```python
from build123d import *

# Parameters (mm, degrees)
SKETCH2_R           = 8.626283366
SKETCH2_R_2         = 2
BOSS_EXTRUDE2_DEPTH = 0.15


with BuildPart() as part:
    # Sketch1 → Revolve1 (revolve)
    with BuildSketch(Plane.XY, mode=Mode.PRIVATE) as revolve1_sk:
        with BuildLine():
            Line((16, 21.11), (16, 20.123658445))
            ThreePointArc((16, 20.123658445), (14.844631277, 19.923379665), (14, 19.11))
            Line((14, 19.11), (14, 13.11))
            ThreePointArc((14, 13.11), (12.760912849, 9.212301981), (9.498573932, 6.745617646))
            ThreePointArc((9.498573932, 6.745617646), (8.602056269, 5.471944767), (7.096455966, 5.073003354))
            ThreePointArc((7.096455966, 5.073003354), (4.361623846, 1.398669209), (0, 0))
            Line((0, 0), (0, 20.221919192))
            ThreePointArc((0, 20.221919192), (5.230275248, 18.600523967), (8.626283366, 14.304964573))
            Line((8.626283366, 14.304964573), (8.626283366, 21.11))
            Line((8.626283366, 21.11), (16, 21.11))
        make_face()
    revolve(revolve1_sk.sketch.rotate(Axis((0, 20.221919192, 0), (0, -1, 0)), 90), axis=Axis((0, 20.221919192, 0), (0, -1, 0)))

    # Sketch2 → Boss-Extrude2 (add)
    with BuildSketch(Plane(origin=(0, 21.11, 0), x_dir=(1, 0, 0), z_dir=(0, 1, 0))):
        with BuildLine():
            Line((-4.400679072, -22.153645833), (-13.285068895, -8.916666667))
            ThreePointArc((-13.285068895, -8.916666667), (-16, 0), (-13.285068895, 8.916666667))
            Line((-13.285068895, 8.916666667), (-4.400679072, 22.153645833))
            ThreePointArc((-4.400679072, 22.153645833), (0, 24.5), (4.400679072, 22.153645833))
            Line((4.400679072, 22.153645833), (13.285068895, 8.916666667))
            ThreePointArc((13.285068895, 8.916666667), (16, 0), (13.285068895, -8.916666667))
            Line((13.285068895, -8.916666667), (4.400679072, -22.153645833))
            ThreePointArc((4.400679072, -22.153645833), (0, -24.5), (-4.400679072, -22.153645833))
        make_face()
        with Locations(Location((0, 0, 0), (0, 0, 270))):
            Circle(SKETCH2_R, mode=Mode.SUBTRACT)
        with Locations(Location((0, -19.2, 0), (0, 0, 270))):
            Circle(SKETCH2_R_2, mode=Mode.SUBTRACT)
        with Locations(Location((0, 19.2, 0), (0, 0, 270))):
            Circle(SKETCH2_R_2, mode=Mode.SUBTRACT)
    extrude(amount=BOSS_EXTRUDE2_DEPTH)


solid = part.part
```
Here's how the part is built. I have some questions about the finished solid (model axes, mm). Round coordinates to 2 decimals unless told otherwise and drop trailing zeros. Order: outer loops, then holes, each group sorted by start corner. A loop starts at its lowest first (then second) coordinate and runs counter-clockwise, first axis right, second up. Notation, with made-up numbers: (-4.75, 20) -> (6.25, 20) arc R21 ccw to (6.25, 28) -> close; hole circle Ø7 at (73.5, 57.25). An arc over 180 degrees is marked (long way). Use a Markdown table: item, result. Add a question column.
(1) I need wall thicknesses on line 1 along Z through (x, y) = (-6, 15.25); line 2 along X through (y, z) = (19.5, 0); line 3 along Z through (x, y) = (-7.5, 15). Which ranges of each line are inside material? Lowest first, please.
(2) For pin 1 Ø1.5 at (x, y) = (11.5, 12.5) entering from +Z; pin 2 Ø15.5 at (x, z) = (0, 0) entering from +Y; pin 3 Ø1 at (y, z) = (13.5, 0.5) entering from +X, each with a flat end and sliding along its axis, tell me the tip position at first contact or that it passes through.
(3) Suppose I cut it at D-D, the plane y = 15.5. Please give me the cut outline in (x, z).
(4) Suppose I cut it at C-C, the plane z = 0. Please give me the cut outline in (x, y).
(5) Suppose I cut it at B-B, the plane x = 0. Please give me the cut outline in (y, z), and give its area (3 significant figures).
(6) Suppose I cut it at A-A, the plane z = 19.2. Please give me the cut outline in (x, y).
(7) If we mould it in two halves opening along Z, with no side actions, what happens to faces 1 (the face through (7, 21.26, -6)), 2 (the face through (-5.249, 17.734, -6.846)), 3 (the face through (12.4, 16.1, 6.5))? For each: released by +Z, released by -Z, zero draft, split by the parting line, or undercut.
Verdict:
| question | item | result |
|---|---|---|
| 1 | line 1 | -12.65 to -6.2, -5.59 to 5.59, 6.2 to 12.65 |
| 1 | line 2 | -14.28 to -8.63, -3.58 to 3.58, 8.63 to 14.28 |
| 1 | line 3 | -11.82 to -4.26, -3.61 to 3.61, 4.26 to 11.82 |
| 2 | pin 1 | z = 8.93 |
| 2 | pin 2 | y = 20.22 |
| 2 | pin 3 | x = 14 |
| 3 | outline | circle Ø28 at (0, 0); circle Ø16.13 at (0, 0); hole circle Ø17.25 at (0, 0) |
| 4 | outline | (-16, 20.12) arc R2 cw to (-14, 19.11) -> (-14, 13.11) arc R6.75 ccw to (-9.5, 6.75) arc R2.28 ccw to (-7.1, 5.07) arc R7.5 ccw to (7.1, 5.07) arc R2.28 ccw to (9.5, 6.75) arc R6.75 ccw to (14, 13.11) -> (14, 19.11) arc R2 cw to (16, 20.12) -> (16, 21.26) -> (8.63, 21.26) -> (8.63, 14.3) arc R9.25 ccw to (-8.63, 14.3) -> (-8.63, 21.26) -> (-16, 21.26) -> close |
| 5 | outline | (5.07, -7.1) arc R2.28 ccw to (6.75, -9.5) arc R6.75 ccw to (13.11, -14) -> (19.11, -14) arc R2 cw to (20.12, -16) -> (21.11, -16) -> (21.11, -17.2) -> (21.26, -17.2) -> (21.26, -8.63) -> (14.3, -8.63) arc R9.25 ccw to (14.3, 8.63) -> (21.26, 8.63) -> (21.26, 17.2) -> (21.11, 17.2) -> (21.11, 16) -> (20.12, 16) arc R2 cw to (19.11, 14) -> (13.11, 14) arc R6.75 ccw to (6.75, 9.5) arc R2.28 ccw to (5.07, 7.1) arc R7.5 ccw to start; (21.11, -24.5) -> (21.26, -24.5) -> (21.26, -21.2) -> (21.11, -21.2) -> close; (21.11, 21.2) -> (21.26, 21.2) -> (21.26, 24.5) -> (21.11, 24.5) -> close |
| 5 | area | 434 mm2 |
| 6 | outline | (-6.38, 21.11) -> (-2, 21.11) -> (-2, 21.26) -> (-6.38, 21.26) -> close; (2, 21.11) -> (6.38, 21.11) -> (6.38, 21.26) -> (2, 21.26) -> close |
| 7 | face 1 | zero draft |
| 7 | face 2 | undercut |
| 7 | face 3 | split by the parting line |
